Part model, mm, in its own coordinate system. A direction names the side the tool comes from. Coordinates: 2 decimals unless noted, no trailing zeros. Write each loop counter-clockwise with the first axis right and the second up, starting at its lowest first coordinate (ties: lowest second). Pieces come first, ordered by that corner, then holes. Notation, with made-up numbers: M 88,21.5 L 105,21.5 A18 ccw 105,39.5 Z; hole C 83.25,89 d6. An arc over 180 degrees is marked long. Use a Markdown table: item, result. Add a question column.
Q1. Pin check, flat tips, straight feed: pin 1 Ø3 at (x, y) = (-22.5, 9) entering from +Z; pin 2 Ø11 at (x, y) = (89.5, 3) entering from +Z; pin 3 Ø5.5 at (x, y) = (-50, -43.5) entering from +Z. Stop position of each tip, or through.
Q2. Wall check: L1, parallel to X at y = -51, z = 1.3; L2, parallel to Y at x = -156, z = 4.45; L3, parallel to Y at x = 0, z = 3.5. Give the ranges that are in metal, low to high. Write a range as from..to.
Q3. Mould opens along X. For faces 3 (the conical face through (-153.6, -13.9, 5.7)), 4 (the flat face through (-96, -51, 8)) say: released by +X, released by -X, zero draft, split by the parting line, or undercut.
Q4. Tool access for faces 1 (the flat face through (-35, -15, 3)), 2 (the cylindrical face through (7, -45, 5)): list every direction of +Z, -Z, +X, -X, +Y, -Y with a clear straight run to the whole face (end or side of a thin tool).
Q5. Slice it at A-A on x = -21.5. Write the cut outline in (y, z), then the cut area to 3 significant figures.
from build123d import *

# Parameters (mm, degrees)
SKETCH1_W                                       = 320
SKETCH1_H                                       = 110
EXTRUDE1_DEPTH                                  = 8
SKETCH2_R                                       = 1.75
CUT_EXTRUDE1_DEPTH                              = 170.378274876
CUT_EXTRUDE2_DEPTH                              = 6
SKETCH7_R                                       = 2.25
CUT_EXTRUDE3_DEPTH                              = 10
SKETCH10_R                                      = 1.5
CUT_EXTRUDE4_DEPTH                              = 10
CSK_FOR_M3_FLAT_HEAD_MACHINE_SCREW3_D           = 3.4
CSK_FOR_M3_FLAT_HEAD_MACHINE_SCREW3_CSINK_D     = 6.3
CSK_FOR_M3_FLAT_HEAD_MACHINE_SCREW3_CSINK_ANGLE = 90
SKETCH13_W                                      = 110
SKETCH13_H                                      = 50
CUT_EXTRUDE5_DEPTH                              = 10
SKETCH14_W                                      = 116
SKETCH14_H                                      = 64
CUT_EXTRUDE6_DEPTH                              = 2
FILLET1_R                                       = 5
SKETCH16_R                                      = 1.65
CUT_EXTRUDE7_DEPTH                              = 10
CSK_FOR_M4_FLAT_HEAD_MACHINE_SCREW1_D           = 4.5
CSK_FOR_M4_FLAT_HEAD_MACHINE_SCREW1_CSINK_D     = 9.4
CSK_FOR_M4_FLAT_HEAD_MACHINE_SCREW1_CSINK_ANGLE = 90


with BuildPart() as part:
    # Sketch1 → Extrude1 (new body)
    with BuildSketch(Plane.XY):
        Rectangle(SKETCH1_W, SKETCH1_H)
    extrude(amount=EXTRUDE1_DEPTH)

    # Sketch2 → Cut-Extrude1 (cut, through all)
    with BuildSketch(Plane.XY.offset(8)):
        with Locations((156, 41)):
            Circle(SKETCH2_R)
        with Locations((156, 14)):
            Circle(SKETCH2_R)
        with Locations(Location((156, -41, 0), (0, 0, 180))):
            Circle(SKETCH2_R)
        with Locations(Location((156, -14, 0), (0, 0, 180))):
            Circle(SKETCH2_R)
        with Locations((-156, -41)):
            Circle(SKETCH2_R)
        with Locations((-156, -14)):
            Circle(SKETCH2_R)
        with Locations(Location((-156, 14, 0), (0, 0, 180))):
            Circle(SKETCH2_R)
        with Locations(Location((-156, 41, 0), (0, 0, 180))):
            Circle(SKETCH2_R)
    extrude(amount=-CUT_EXTRUDE1_DEPTH, mode=Mode.SUBTRACT)

    # Sketch6 → Cut-Extrude2 (cut)
    with BuildSketch(Plane.XY.offset(8)):
        with BuildLine():
            Line((150, 40), (150, -40))
            ThreePointArc((150, -40), (145, -45), (140, -40))
            Line((140, -40), (140, 40))
            ThreePointArc((140, 40), (145, 45), (150, 40))
        make_face()
        with BuildLine():
            Line((136.19047619, 40), (136.19047619, -40))
            ThreePointArc((136.19047619, -40), (131.19047619, -45), (126.19047619, -40))
            Line((126.19047619, -40), (126.19047619, 40))
            ThreePointArc((126.19047619, 40), (131.19047619, 45), (136.19047619, 40))
        make_face()
        with BuildLine():
            Line((122.380952381, 40), (122.380952381, -40))
            ThreePointArc((122.380952381, -40), (117.380952381, -45), (112.380952381, -40))
            Line((112.380952381, -40), (112.380952381, 40))
            ThreePointArc((112.380952381, 40), (117.380952381, 45), (122.380952381, 40))
        make_face()
        with BuildLine():
            Line((108.571428571, 40), (108.571428571, -40))
            ThreePointArc((108.571428571, -40), (103.571428571, -45), (98.571428571, -40))
            Line((98.571428571, -40), (98.571428571, 40))
            ThreePointArc((98.571428571, 40), (103.571428571, 45), (108.571428571, 40))
        make_face()
        with BuildLine():
            Line((94.761904762, 40), (94.761904762, -40))
            ThreePointArc((94.761904762, -40), (89.761904762, -45), (84.761904762, -40))
            Line((84.761904762, -40), (84.761904762, 40))
            ThreePointArc((84.761904762, 40), (89.761904762, 45), (94.761904762, 40))
        make_face()
        with BuildLine():
            Line((80.952380952, 40), (80.952380952, -40))
            ThreePointArc((80.952380952, -40), (75.952380952, -45), (70.952380952, -40))
            Line((70.952380952, -40), (70.952380952, 40))
            ThreePointArc((70.952380952, 40), (75.952380952, 45), (80.952380952, 40))
        make_face()
        with BuildLine():
            Line((67.142857143, 40), (67.142857143, -40))
            ThreePointArc((67.142857143, -40), (62.142857143, -45), (57.142857143, -40))
            Line((57.142857143, -40), (57.142857143, 40))
            ThreePointArc((57.142857143, 40), (62.142857143, 45), (67.142857143, 40))
        make_face()
        with BuildLine():
            Line((53.333333333, 40), (53.333333333, -40))
            ThreePointArc((53.333333333, -40), (48.333333333, -45), (43.333333333, -40))
            Line((43.333333333, -40), (43.333333333, 40))
            ThreePointArc((43.333333333, 40), (48.333333333, 45), (53.333333333, 40))
        make_face()
        with BuildLine():
            Line((39.523809524, 40), (39.523809524, -40))
            ThreePointArc((39.523809524, -40), (34.523809524, -45), (29.523809524, -40))
            Line((29.523809524, -40), (29.523809524, 40))
            ThreePointArc((29.523809524, 40), (34.523809524, 45), (39.523809524, 40))
        make_face()
        with BuildLine():
            Line((25.714285714, 40), (25.714285714, -40))
            ThreePointArc((25.714285714, -40), (20.714285714, -45), (15.714285714, -40))
            Line((15.714285714, -40), (15.714285714, 40))
            ThreePointArc((15.714285714, 40), (20.714285714, 45), (25.714285714, 40))
        make_face()
        with BuildLine():
            Line((11.904761905, 40), (11.904761905, -40))
            ThreePointArc((11.904761905, -40), (6.904761905, -45), (1.904761905, -40))
            Line((1.904761905, -40), (1.904761905, 40))
            ThreePointArc((1.904761905, 40), (6.904761905, 45), (11.904761905, 40))
        make_face()
        with BuildLine():
            Line((-1.904761905, 40), (-1.904761905, -40))
            ThreePointArc((-1.904761905, -40), (-6.904761905, -45), (-11.904761905, -40))
            Line((-11.904761905, -40), (-11.904761905, 40))
            ThreePointArc((-11.904761905, 40), (-6.904761905, 45), (-1.904761905, 40))
        make_face()
        with BuildLine():
            Line((-15.714285714, 40), (-15.714285714, -40))
            ThreePointArc((-15.714285714, -40), (-20.714285714, -45), (-25.714285714, -40))
            Line((-25.714285714, -40), (-25.714285714, 40))
            ThreePointArc((-25.714285714, 40), (-20.714285714, 45), (-15.714285714, 40))
        make_face()
    extrude(amount=-CUT_EXTRUDE2_DEPTH, mode=Mode.SUBTRACT)

    # Sketch7 → Cut-Extrude3 (cut)
    with BuildSketch(Plane.XY.offset(8)):
        with Locations((-64, -51)):
            Circle(SKETCH7_R)
        with Locations((0, -51)):
            Circle(SKETCH7_R)
        with Locations((64, -51)):
            Circle(SKETCH7_R)
        with Locations((-128, -51)):
            Circle(SKETCH7_R)
        with Locations((128, -51)):
            Circle(SKETCH7_R)
    extrude(amount=-CUT_EXTRUDE3_DEPTH, mode=Mode.SUBTRACT)

    # Sketch10 → Cut-Extrude4 (cut)
    with BuildSketch(Plane.XY.offset(8)):
        with Locations((101.5, 52)):
            Circle(SKETCH10_R)
        with Locations((-101.5, 52)):
            Circle(SKETCH10_R)
    extrude(amount=-CUT_EXTRUDE4_DEPTH, mode=Mode.SUBTRACT)

    # CSK for M3 Flat Head Machine Screw3 (through all)
    with Locations(Plane.XY.offset(8)):
        with Locations((-101.5, 52), (101.5, 52)):
            CounterSinkHole(CSK_FOR_M3_FLAT_HEAD_MACHINE_SCREW3_D / 2, CSK_FOR_M3_FLAT_HEAD_MACHINE_SCREW3_CSINK_D / 2, counter_sink_angle=CSK_FOR_M3_FLAT_HEAD_MACHINE_SCREW3_CSINK_ANGLE)

    # Sketch13 → Cut-Extrude5 (cut)
    with BuildSketch(Plane.XY.offset(8)):
        with Locations((-90, -15)):
            Rectangle(SKETCH13_W, SKETCH13_H)
    extrude(amount=-CUT_EXTRUDE5_DEPTH, mode=Mode.SUBTRACT)

    # Sketch14 → Cut-Extrude6 (cut)
    with BuildSketch(Plane.XY.offset(8)):
        with Locations((-90, -15)):
            Rectangle(SKETCH14_W, SKETCH14_H)
    extrude(amount=-CUT_EXTRUDE6_DEPTH, mode=Mode.SUBTRACT)

    # Fillet1
    fillet1_edges = [part.edges().sort_by_distance(p)[0] for p in [
        (-145, -40, 3),
        (-145, 10, 3),
        (-35, 10, 3),
        (-35, -40, 3),
        (-148, -47, 7),
        (-148, 17, 7),
        (-32, 17, 7),
        (-32, -47, 7),
    ]]
    fillet(fillet1_edges, radius=FILLET1_R)

    # Sketch16 → Cut-Extrude7 (cut)
    with BuildSketch(Plane.XY.offset(6)):
        with Locations((-130, -43.5)):
            Circle(SKETCH16_R)
        with Locations((-50, -43.5)):
            Circle(SKETCH16_R)
        with Locations((-50, 13.5)):
            Circle(SKETCH16_R)
        with Locations((-130, 13.5)):
            Circle(SKETCH16_R)
    extrude(amount=-CUT_EXTRUDE7_DEPTH, mode=Mode.SUBTRACT)

    # CSK for M4 Flat Head Machine Screw1 (through all)
    with Locations(Plane.XY.offset(8)):
        with Locations((156, 41), (156, 14), (156, -41), (-156, -41), (-156, -14), (-156, 14), (-156, 41), (156, -14), (-128, -51), (-64, -51), (0, -51), (64, -51), (128, -51)):
            CounterSinkHole(CSK_FOR_M4_FLAT_HEAD_MACHINE_SCREW1_D / 2, CSK_FOR_M4_FLAT_HEAD_MACHINE_SCREW1_CSINK_D / 2, counter_sink_angle=CSK_FOR_M4_FLAT_HEAD_MACHINE_SCREW1_CSINK_ANGLE)


solid = part.part
Recorded:
| question | item | result |
|---|---|---|
| 1 | pin 1 | z = 2 |
| 1 | pin 2 | z = 8 |
| 1 | pin 3 | z = 6 |
| 2 | L1 | -160..-130.25, -125.75..-66.25, -61.75..-2.25, 2.25..61.75, 66.25..125.75, 130.25..160 |
| 2 | L2 | -55..-43.25, -38.75..-16.25, -11.75..11.75, 16.25..38.75, 43.25..55 |
| 2 | L3 | -55..-53.25, -48.75..55 |
| 3 | face 3 | undercut |
| 3 | face 4 | zero draft |
| 4 | face 1 | +Z, -Z |
| 4 | face 2 | +Z |
| 5 | outline | M -55,0 L 55,0 L 55,8 L 44.94,8 L 44.94,2 L -44.94,2 L -44.94,8 L -55,8 Z |
| 5 | area | 341 mm² |
